Geometry check sheet. Reference: the model listing, model coordinates, mm. A direction names the side the tool comes from. Round coordinates to 2 decimals unless told otherwise and drop trailing zeros. Order: outer loops, then holes, each group sorted by start corner. A loop starts at its lowest first (then second) coordinate and runs counter-clockwise, first axis right, second up. Notation, with made-up numbers: M 74.5,-32.5 L 118.5,-32.5 A13 ccw 118.5,-15.5 Z; hole C 74,8.25 d2. An arc over 180 degrees is marked long. Return JSON: item names as keys, results as strings. Group by question number.
```python
from build123d import *
from OCP.BRepFilletAPI import BRepFilletAPI_MakeFillet

# Parameters (mm, degrees)
BOSS_EXTRUDE1_DEPTH     = 1
CUT_EXTRUDE1_DEPTH      = 72.854018677
CUT_EXTRUDE2_DEPTH      = 72.854018677
CUT_EXTRUDE2_DEPTH_BACK = 72.854018677
SKETCH2_R               = 2
FILLET1_R               = 3
FILLET2_R               = 3
FILLET3_R1              = 5
FILLET3_R2              = 3
FILLET4_R               = 1
LPATTERN1_COUNT         = 4
LPATTERN1_PITCH         = 12
FILLET4_OF_LPATTERN1_R  = 1


with BuildPart() as part:
    # Sketch1 → Boss-Extrude1 (new, symmetric)
    with BuildSketch(Plane(origin=(0, 0, 0), x_dir=(1, 0, 0), z_dir=(0, 1, 0))):
        Polygon((-6, 56), (6, 71), (6, 16), (11, 12), (11, 6), (7.5, 3), (2.5, 3), (2.5, 0), (-2.5, 0), (-2.5, 3), (-7.5, 3), (-11, 6), (-11, 12), (-6, 16), align=None)
    extrude(amount=BOSS_EXTRUDE1_DEPTH, both=True)

    # Sketch1<3> → Cut-Extrude1 (cut, symmetric)
    with BuildSketch(Plane(origin=(0, 0, 0), x_dir=(1, 0, 0), z_dir=(0, 1, 0))):
        Polygon((3, 61.25), (-3, 53.75), (-3, 47.75), (3, 55.25), align=None)
    cut_extrude1 = extrude(amount=CUT_EXTRUDE1_DEPTH, both=True, mode=Mode.SUBTRACT)

    # Sketch2 → Cut-Extrude2 (cut, two sides: drawn at the far end of the back side and taken through both)
    with BuildSketch(Plane(origin=(0, 0, 0), x_dir=(1, 0, 0), z_dir=(0, 1, 0)).offset(-CUT_EXTRUDE2_DEPTH_BACK)):
        with Locations(Location((-6, 9, 0), (0, 0, 270))):
            Circle(SKETCH2_R)
        with Locations(Location((6, 9, 0), (0, 0, 270))):
            Circle(SKETCH2_R)
    extrude(amount=CUT_EXTRUDE2_DEPTH + CUT_EXTRUDE2_DEPTH_BACK, mode=Mode.SUBTRACT)

    # Fillet1
    fillet1_edges = [part.edges().sort_by_distance(p)[0] for p in [
        (2.5, 0, -3),
        (-2.5, 0, -3),
    ]]
    fillet(fillet1_edges, radius=FILLET1_R - 0.0001)  # a hair under: the kernel refuses the full size

    # Fillet2
    fillet2_edges = [part.edges().sort_by_distance(p)[0] for p in [
        (-6, 0, -16),
        (-11, 0, -12),
        (-11, 0, -6),
        (-7.5, 0, -3),
        (7.5, 0, -3),
        (11, 0, -6),
        (11, 0, -12),
        (6, 0, -16),
    ]]
    fillet(fillet2_edges, radius=FILLET2_R)

    # Fillet3: one fillet with a radius per group of edges: ONE call of the kernel's fillet builder (fillet() takes one radius for all edges)
    fillet3_edges_1 = [part.edges().sort_by_distance(p)[0] for p in [
        (-6, 0, -56),
    ]]
    fillet3_edges_2 = [part.edges().sort_by_distance(p)[0] for p in [
        (6, 0, -71),
    ]]
    fillet3 = BRepFilletAPI_MakeFillet(part.part.solid().wrapped)
    for e in fillet3_edges_1:
        fillet3.Add(FILLET3_R1, e.wrapped)
    for e in fillet3_edges_2:
        fillet3.Add(FILLET3_R2, e.wrapped)
    add(Compound.cast(fillet3.Shape()), mode=Mode.REPLACE)

    # Fillet4
    fillet4_edges = [part.edges().sort_by_distance(p)[0] for p in [
        (-3, 0, -47.75),
        (-3, 0, -53.75),
        (3, 0, -61.25),
        (3, 0, -55.25),
    ]]
    fillet(fillet4_edges, radius=FILLET4_R)

    # LPattern1: Cut-Extrude1 ×4
    with Locations(*[(0, 0, i * LPATTERN1_PITCH) for i in range(1, LPATTERN1_COUNT)]):
        add(cut_extrude1, mode=Mode.SUBTRACT)

    # Fillet4 of LPattern1
    fillet4_of_lpattern1_edges = [part.edges().sort_by_distance(p)[0] for p in [
        (-3, 0, -35.75),
        (-3, 0, -41.75),
        (3, 0, -49.25),
        (3, 0, -43.25),
        (-3, 0, -23.75),
        (-3, 0, -29.75),
        (3, 0, -37.25),
        (3, 0, -31.25),
        (-3, 0, -11.75),
        (-3, 0, -17.75),
        (3, 0, -25.25),
        (3, 0, -19.25),
    ]]
    fillet(fillet4_of_lpattern1_edges, radius=FILLET4_OF_LPATTERN1_R)


solid = part.part
```
Q1. Section check B-B on y = -0.5. Count the separate pieces of the cut face and the enclosed holes in it, plus the area to 3 significant figures.
Q2. Section check C-C on z = -61. Record the cut outline in (x, y), plus the area to 3 significant figures.
Q3. Section check D-D on z = -25. Record the cut outline in (x, y).
Q4. Depth check by flat-ended pin: pin 1 Ø0.6 at (y, z) = (0, -44.5) entering from -X; pin 2 Ø3.5 at (x, z) = (-6, -9) entering from -Y; pin 3 Ø1 at (y, z) = (-0.5, -57) entering from -X; pin 4 Ø0.6 at (y, z) = (0, -47) entering from +X. Enter the tip coordinate at first touch or a pass-through.
Q5. Set-up check for faces 5 (the face through (3, 0, -45)), 6 (the face through (-3.4, -0.01, -2.14)): record each of +Z, -Z, +X, -X, +Y, -Y from which the full face is reachable in a straight line by a thin tool's end or side.
Q6. Release check for a two-part mould opening along X. For faces 1 (the face through (-8.5, 0, -14)), 2 (the face through (10.72, -0.01, -6.11)), 3 (the face through (-2.31, 0.01, -37.65)), 4 (the face through (-0.75, 0.01, -20.56)) record: +X half, -X half, draft (parallel to the pull), parting line (faces both ways), or undercut.
Q7. Material ranges on line 1 along X through (y, z) = (0.2, -9); line 2 along Z through (x, y) = (-1.75, 0.95); line 3 along Z through (x, y) = (2.25, 0.7), recorded low to high.
Q8. Section check A-A on z = -9. Record the cut outline in (x, y), plus the area to 3 significant figures.
Geometry check:
{
 "1": {"separate pieces": "1", "enclosed holes": "6", "area": "673 mm^2"},
 "2": {"outline": "M -2,-1 L 6,-1 L 6,1 L -2,1 Z", "area": "16.0 mm^2"},
 "3": {"outline": "M -6,-1 L 6,-1 L 6,1 L -6,1 Z"},
 "4": {"pin 1": "stops at x = -6", "pin 2": "passes through", "pin 3": "stops at x = -5.46", "pin 4": "stops at x = 6"},
 "5": {"face 5": "+Y, -Y", "face 6": "+Z, -X, +Y, -Y"},
 "6": {"face 1": "-X half", "face 2": "+X half", "face 3": "undercut", "face 4": "undercut"},
 "7": {"line 1": "x = -11 to -8, -4 to 4, 8 to 11", "line 2": "z = -61.31 to -55.31, -49.63 to -43.31, -37.63 to -31.31, -25.63 to -19.31, -13.63 to 0", "line 3": "z = -65.35 to -59.37, -54.31 to -47.37, -42.31 to -35.37, -30.31 to -23.37, -18.31 to 0"},
 "8": {"outline": "M -11,-1 L -8,-1 L -8,1 L -11,1 Z; M -4,-1 L 4,-1 L 4,1 L -4,1 Z; M 8,-1 L 11,-1 L 11,1 L 8,1 Z", "area": "28.0 mm^2"}
}
